Design review of the part built by this model. Coordinates are the model's own, in mm. A direction names the side the tool comes from. Coordinates: 2 decimals unless noted, no trailing zeros. Loops run counter-clockwise (first coordinate to the right, second up) from the corner with the lowest first, then second, coordinate; pieces in that order, holes last. Notation, with made-up numbers: (-2.75, 11.5) -> (37.25, 11.5) arc R7 ccw to (37.25, 15.5) -> close; hole circle Ø2 at (-7, 7.25). An arc over 180 degrees is marked (long way). Answer in a Markdown table with one row per item.
```python
from build123d import *

# Parameters (mm, degrees)
SKETCH1_W           = 20
SKETCH1_H           = 20
BOSS_EXTRUDE2_DEPTH = 160.4
SKETCH1_3_W         = 20
SKETCH1_3_H         = 20
BOSS_EXTRUDE3_DEPTH = 28.575


with BuildPart() as part:
    # Sketch1 → Boss-Extrude2 (new body)
    with BuildSketch(Plane(origin=(0, 0, 0), x_dir=(1, 0, 0), z_dir=(0, 1, 0))):
        Rectangle(SKETCH1_W, SKETCH1_H)
    extrude(amount=BOSS_EXTRUDE2_DEPTH)

    # Sketch1_3 → Boss-Extrude3 (add)
    with BuildSketch(Plane(origin=(0, 0, 0), x_dir=(1, 0, 0), z_dir=(0, 1, 0))):
        with BuildLine():
            Line((10, -10), (-10, -10))
            ThreePointArc((-10, -10), (0, -14.142135624), (10, -10))
        make_face()
        with BuildLine():
            ThreePointArc((-10, 10), (-14.142135624, 0), (-10, -10))
            Line((-10, -10), (-10, 10))
        make_face()
        Rectangle(SKETCH1_3_W, SKETCH1_3_H)
        with BuildLine():
            Line((10, 10), (10, -10))
            ThreePointArc((10, -10), (13.065629649, -5.411961001), (14.142135624, 0))
            ThreePointArc((14.142135624, 0), (13.065629649, 5.411961001), (10, 10))
        make_face()
        with BuildLine():
            ThreePointArc((10, 10), (0, 14.142135624), (-10, 10))
            Line((-10, 10), (10, 10))
        make_face()
    extrude(amount=-BOSS_EXTRUDE3_DEPTH)


solid = part.part
```
(1) To check wall thickness, follow probe 1 along Z at (x, y) = (-1, 8); probe 2 along Y at (x, z) = (11.75, -1.75) (3 decimals). State the ranges of each line that lie inside material, in increasing order.
Evaluation:
| item | result |
|---|---|
| probe 1 | z = -10 to 10 |
| probe 2 | y = -28.575 to 0 |
(2) For pin 1 (4.5 mm diameter, centred on x = 3.5, z = 12.5, fed in from +Y); pin 2 (4 mm diameter, centred on y = 56.5, z = -4.5, fed in from -X); pin 3 (8 mm diameter, centred on y = 35.5, z = 4.5, fed in from +X), all flat-tipped, find the tip position at first contact; note any pin that passes through.
Evaluation:
| item | result |
|---|---|
| pin 1 | stops at y = 0 |
| pin 2 | stops at x = -10 |
| pin 3 | stops at x = 10 |
(3) Take a section at D-D on x = 12. Give the boundary of the cut face in (y, z) (3 decimals).
Evaluation:
| item | result |
|---|---|
| outline | (-28.575, -7.483) -> (0, -7.483) -> (0, 7.483) -> (-28.575, 7.483) -> close |
(4) Tool access review of faces 1 (the flat face through (0, 160.4, 0)), 2 (the flat face through (0, 79, 10)), 3 (the flat face through (-10, 79, 0)), 4 (the flat face through (0, 0, -12)), 5 (the flat face through (10, 79, 0)): name each direction out of +Z, -Z, +X, -X, +Y, -Y from which nothing blocks a thin tool from reaching the whole face with its end or side.
Evaluation:
| item | result |
|---|---|
| face 1 | +Z, -Z, +X, -X, +Y |
| face 2 | +Z, +X, -X, +Y |
| face 3 | +Z, -Z, -X, +Y |
| face 4 | -Z, +X, -X, +Y |
| face 5 | +Z, -Z, +X, +Y |
(5) Take a section at B-B on z = 3.5. Give the boundary of the cut face in (x, y) (3 decimals).
Evaluation:
| item | result |
|---|---|
| outline | (-13.702, -28.575) -> (13.702, -28.575) -> (13.702, 0) -> (10, 0) -> (10, 160.4) -> (-10, 160.4) -> (-10, 0) -> (-13.702, 0) -> close |
(6) Take a section at C-C on y = 123. Give the boundary of the cut face in (x, z), and give its area (3 significant figures).
Evaluation:
| item | result |
|---|---|
| outline | (-10, -10) -> (10, -10) -> (10, 10) -> (-10, 10) -> close |
| area | 400 mm² |
(7) Take a section at A-A on x = -6.25. Give the boundary of the cut face in (y, z) (3 decimals), and give its area (3 significant figures).
Evaluation:
| item | result |
|---|---|
| outline | (-28.575, -12.686) -> (0, -12.686) -> (0, -10) -> (160.4, -10) -> (160.4, 10) -> (0, 10) -> (0, 12.686) -> (-28.575, 12.686) -> close |
| area | 3,930 mm² |
